from build123d import *

# Parameters (mm, degrees)
SKETCH_1_W          = 225
SKETCH_1_H          = 20
EXTRUDE_1_DEPTH     = 2
SKETCH_2_R          = 2.6
CUT_EXTRUDE_1_DEPTH = 113.961276551
FILLET_1_R          = 5


with BuildPart() as part:
    # 草图1 → 凸台-拉伸1 (new body)
    with BuildSketch(Plane.XY):
        Rectangle(SKETCH_1_W, SKETCH_1_H)
    extrude(amount=EXTRUDE_1_DEPTH)

    # 草图2 → 切除-拉伸1 (cut, through all)
    with BuildSketch(Plane(origin=(0, 0, 0), x_dir=(-1, 0, 0), z_dir=(0, 0, -1))):
        with Locations((95, 0)):
            Circle(SKETCH_2_R)
        with Locations((75, 0)):
            Circle(SKETCH_2_R)
        with Locations((30, 0)):
            Circle(SKETCH_2_R)
        with Locations((20, 0)):
            Circle(SKETCH_2_R)
        with Locations((10, 0)):
            Circle(SKETCH_2_R)
        with Locations((-35, 0)):
            Circle(SKETCH_2_R)
        with Locations((-55, 0)):
            Circle(SKETCH_2_R)
        with Locations((-85, 0)):
            Circle(SKETCH_2_R)
    extrude(amount=-CUT_EXTRUDE_1_DEPTH, mode=Mode.SUBTRACT)

    # 圆角1
    fillet_1_edges = [part.edges().sort_by_distance(p)[0] for p in [
        (112.5, -10, 1),
        (-112.5, -10, 1),
        (-112.5, 10, 1),
        (112.5, 10, 1),
    ]]
    fillet(fillet_1_edges, radius=FILLET_1_R)


solid = part.part
CAD build for the part. Positions are in the model's coordinates, mm. Round coordinates to 2 decimals unless told otherwise and drop trailing zeros. Order: outer loops, then holes, each group sorted by start corner. A loop starts at its lowest first (then second) coordinate and runs counter-clockwise, first axis right, second up. Notation, with made-up numbers: (36, 37) -> (71, 37) arc R12 cw to (71, 56) -> close; hole circle Ø2 at (3, -25.5). An arc over 180 degrees is marked (long way). Write item = value, one per line. Start each with the question number.
(1) Cut at A-A, the plane x = -95. List the corners of the cut face in (y, z), then the cut area to 3 significant figures.
(2) Pull direction Y, two halves, no side cores. Call faces 1 (the cylindrical face through (-111.07, -8.5, 1.01)), 2 (the cylindrical face through (37.6, 0.1, 1)), 3 (the cylindrical face through (111, 8.57, 1.01)): released by +Y, released by -Y, zero draft, split by the parting line, or undercut.
(3) Probe line 1 (Y direction, x = -20, z = 1.05); line 2 (X direction, y = 8.5, z = 1.3); line 3 (X direction, y = -7.5, z = 0.1). List the from-to ranges inside material, lowest first. Write a range as [from, to].
(4) Pin check, flat tip, straight feed: P1, Ø3, axis at x = -75, y = 0, coming from the +Z side. Stop position of the tip, or through.
(5) Cut at B-B, the plane z = 1.6. State how many separate pieces and enclosed holes the cut face has, then the cut area to 3 significant figures.
Model answer:
q1.outline = (-10, 0) -> (-2.6, 0) -> (-2.6, 2) -> (-10, 2) -> close; (2.6, 0) -> (10, 0) -> (10, 2) -> (2.6, 2) -> close
q1.area = 29.6 mm2
q2.face_1 = released by -Y
q2.face_2 = undercut
q2.face_3 = released by +Y
q3.line_1 = [-10, -2.6], [2.6, 10]
q3.line_2 = [-111.07, 111.07]
q3.line_3 = [-111.83, 111.83]
q4.P1 = through
q5.separate_pieces = 1
q5.enclosed_holes = 8
q5.area = 4,310 mm2
